Verification items for this drawing (mm, ordinates from the low corner). Give positions to 0.01 mm unless a question says otherwise; leave off trailing zeros. Write each loop counter-clockwise with the first axis right and the second up, starting at its lowest first coordinate (ties: lowest second). Pieces come first, ordered by that corner, then holes. Notation, with made-up numbers: (32, -14.75) -> (77, -14.75) arc R15 cw to (77, 12.25) -> close; hole circle Ø6 at (38, -6.75). An arc over 180 degrees is marked (long way). Write item = value, one per line.
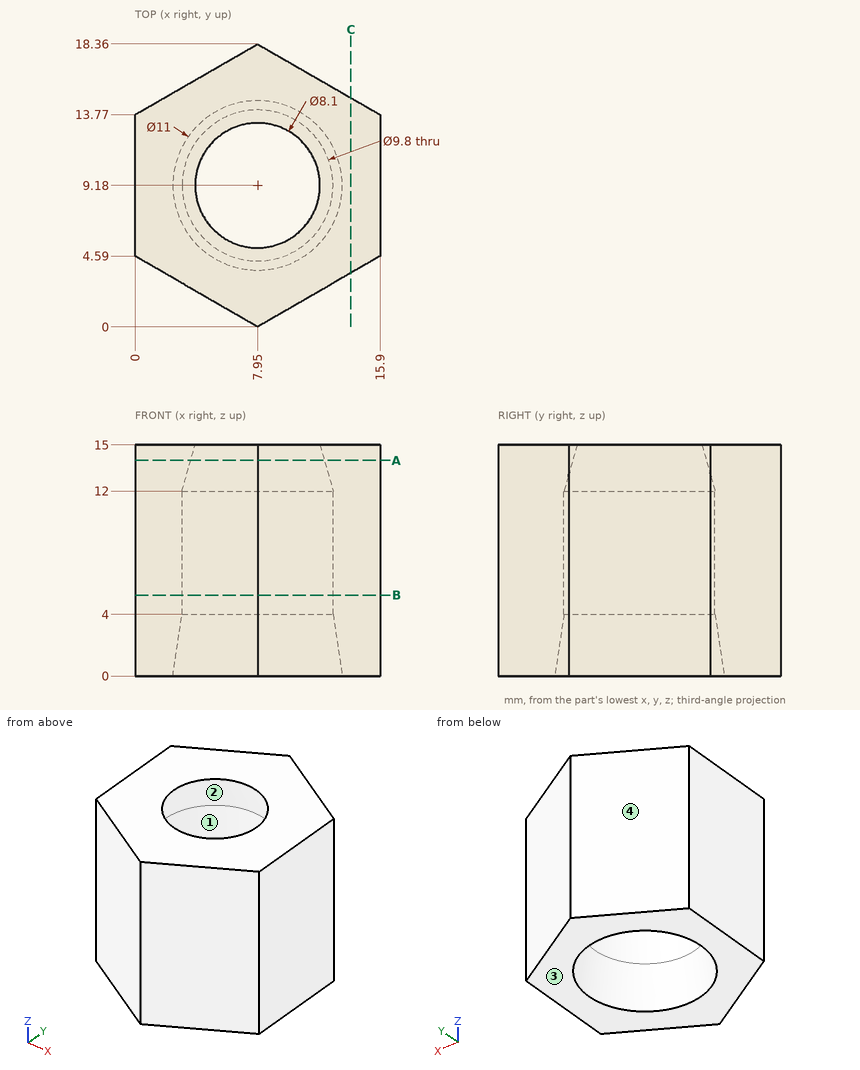
Item 1: Go/stop test with flat-tipped pins: P1, Ø1, axis at y = 15, z = 6, coming from the -X side (1 decimal); P2, Ø4, axis at x = 5, z = 13, coming from the -Y side; P3, Ø4, axis at x = 9.5, z = 6.5, coming from the +Y side. Record where each tip stops, or that it passes through.
Response values:
P1 = 1.3
P2 = 0.55
P3 = 18.36
Item 2: Mould release check, pull along X, two halves, no side actions. Record for the marked faces 1, 2, 3 and 4: +X half, -X half, draft (parallel to the pull), parting line (faces both ways), or undercut.
Response values:
face_1 = undercut
face_2 = undercut
face_3 = draft
face_4 = -X half
Item 3: Sectioned sample at B-B on z = 5.25. Record the cut outline in (x, y).
Response values:
outline = (0, 4.59) -> (7.95, 0) -> (15.9, 4.59) -> (15.9, 13.77) -> (7.95, 18.36) -> (0, 13.77) -> close; hole circle Ø9.8 at (7.95, 9.18)
Item 4: Sectioned sample at A-A on z = 14. Record the cut outline in (x, y).
Response values:
outline = (0, 4.59) -> (7.95, 0) -> (15.9, 4.59) -> (15.9, 13.77) -> (7.95, 18.36) -> (0, 13.77) -> close; hole circle Ø8.67 at (7.95, 9.18)
Item 5: Sectioned sample at C-C on x = 14. Record the cut outline in (y, z).
Response values:
outline = (3.49, 0) -> (14.87, 0) -> (14.87, 15) -> (3.49, 15) -> close
Item 6: Material ranges on line 1 (X direction, y = 7, z = 13.5); line 2 (Y direction, x = 4.5, z = 4.5); line 3 (Y direction, x = 7.75, z = 4) (1 decimal), recorded low to high.
Response values:
line_1 = 0 to 4.04, 11.86 to 15.9
line_2 = 1.99 to 5.7, 12.66 to 16.37
line_3 = 0.1 to 4.3, 14.1 to 18.2
